from build123d import *

# Parameters (mm, degrees)
PAD_DEPTH       = 3
SKETCH001_R     = 4
PAD001_DEPTH    = 5
SKETCH002_R     = 4.5
POCKET_DEPTH    = 8.001
SKETCH003_R     = 1
POCKET001_DEPTH = 5


with BuildPart() as part:
    # Sketch → Pad (new body)
    with BuildSketch(Plane.XZ):
        with BuildLine():
            ThreePointArc((6, 40), (1.757359, 38.242641), (0, 34))
            Line((0, 6), (0, 34))
            ThreePointArc((0, 6), (1.757359, 1.757359), (6, 0))
            Line((144, 0), (6, 0))
            ThreePointArc((144, 0), (148.242641, 1.757359), (150, 6))
            Line((150, 34), (150, 6))
            ThreePointArc((150, 34), (148.242641, 38.242641), (144, 40))
            Line((6, 40), (144, 40))
        make_face()
    extrude(amount=PAD_DEPTH)

    # Sketch001 (on Face9 of Pad) → Pad001 (join)
    with BuildSketch(Plane(origin=(0, 0, 0), x_dir=(1, 0, 0), z_dir=(0, 1, 0))):
        with Locations((8, -8)):
            Circle(SKETCH001_R)
        with Locations((8, -32)):
            Circle(SKETCH001_R)
        with Locations((142, -8)):
            Circle(SKETCH001_R)
        with Locations((142, -32)):
            Circle(SKETCH001_R)
        with Locations((75, -8)):
            Circle(SKETCH001_R)
        with Locations((75, -32)):
            Circle(SKETCH001_R)
    extrude(amount=PAD001_DEPTH)

    # Sketch002 (on Face5 of Pad001) → Pocket (cut, through all)
    with BuildSketch(Plane.XZ.offset(3)):
        with Locations((21.2, 20)):
            Circle(SKETCH002_R)
        with Locations((75, 20)):
            Circle(SKETCH002_R)
        with Locations((128.8, 20)):
            Circle(SKETCH002_R)
    extrude(amount=-POCKET_DEPTH, mode=Mode.SUBTRACT)

    # Sketch003 (on Face25 of Pocket) → Pocket001 (cut)
    with BuildSketch(Plane(origin=(0, 5, 0), x_dir=(1, 0, 0), z_dir=(0, 1, 0))):
        with Locations((8, -8)):
            Circle(SKETCH003_R)
        with Locations((8, -32)):
            Circle(SKETCH003_R)
        with Locations((75, -32)):
            Circle(SKETCH003_R)
        with Locations((142, -32)):
            Circle(SKETCH003_R)
        with Locations((75, -8)):
            Circle(SKETCH003_R)
        with Locations((142, -8)):
            Circle(SKETCH003_R)
    extrude(amount=-POCKET001_DEPTH, mode=Mode.SUBTRACT)


solid = part.part
Design review of the part built by this model. Coordinates are the model's own, in mm. A direction names the side the tool comes from. Round coordinates to 2 decimals unless told otherwise and drop trailing zeros. Loops run counter-clockwise (first coordinate to the right, second up) from the corner with the lowest first, then second, coordinate; pieces in that order, holes last. Notation, with made-up numbers: (41.5, 38.25) - (54.5, 38.25) arc R16 cw to (54.5, 51.25) - close; hole circle Ø2 at (13, -23). An arc over 180 degrees is marked (long way). One line per question, with ' | ' between items.
1. We need section D-D, the plane z = 14. State the section outline as (x, y) points.
Results are:
outline: (0, -3) - (150, -3) - (150, 0) - (0, 0) - close
2. We need section A-A, the plane y = 3. State how many separate pieces and enclosed holes the cut face has, and give its area (3 significant figures).
Results are:
separate pieces: 6 | enclosed holes: 6 | area: 283 mm²
3. Clearance check with flat-ended pins moving along their axes: P1, Ø1, axis at x = 8, z = 8, coming from the +Y side; P2, Ø7, axis at x = 21.2, z = 20, coming from the +Y side. State where each tip first meets the part, or that it passes through.
Results are:
P1: stops at y = 0 | P2: passes through
4. For faces 4 (the face through (7.479, 2.465, 28.034)), 5 (the face through (9, 5, 33)), list the 3-axis set-ups (+Z, -Z, +X, -X, +Y, -Y) from which the entire face can be reached by the end or side of a thin tool; tool diameter is ignored.
Results are:
face 4: +Y | face 5: +Z, -Z, +X, -X, +Y
5. Draft analysis for pull direction X (two halves, no side actions). For faces 1 (the face through (148.196, -1.479, 1.711)), 2 (the face through (76, 5, 33)), 3 (the face through (74.479, 2.465, 28.034)), state which applies: released by +X, released by -X, zero draft, split by the parting line, or undercut.
Results are:
face 1: released by +X | face 2: zero draft | face 3: undercut
6. We need section B-B, the plane z = 20. State the section outline as (x, y) points.
Results are:
outline: (0, -3) - (16.7, -3) - (16.7, 0) - (0, 0) - close; (25.7, -3) - (70.5, -3) - (70.5, 0) - (25.7, 0) - close; (79.5, -3) - (124.3, -3) - (124.3, 0) - (79.5, 0) - close; (133.3, -3) - (150, -3) - (150, 0) - (133.3, 0) - close
7. We need section C-C, the plane x = 20.5. State the section outline as (y, z) points, and give its area (3 significant figures).
Results are:
outline: (-3, 0) - (0, 0) - (0, 15.55) - (-3, 15.55) - close; (-3, 24.45) - (0, 24.45) - (0, 40) - (-3, 40) - close | area: 93.3 mm²
8. For L1, parallel to Z at x = 75, y = 3.55; L2, parallel to X at y = 2.8, z = 32; L3, parallel to Z at x = 128.8, y = -1.6, list the stretches that pass through material, from the lowest coordinate up. Write a range as [from, to].
Results are:
L1: z = [4, 7], [9, 12], [28, 31], [33, 36] | L2: x = [4, 7], [9, 12], [71, 74], [76, 79], [138, 141], [143, 146] | L3: z = [0, 15.5], [24.5, 40]
